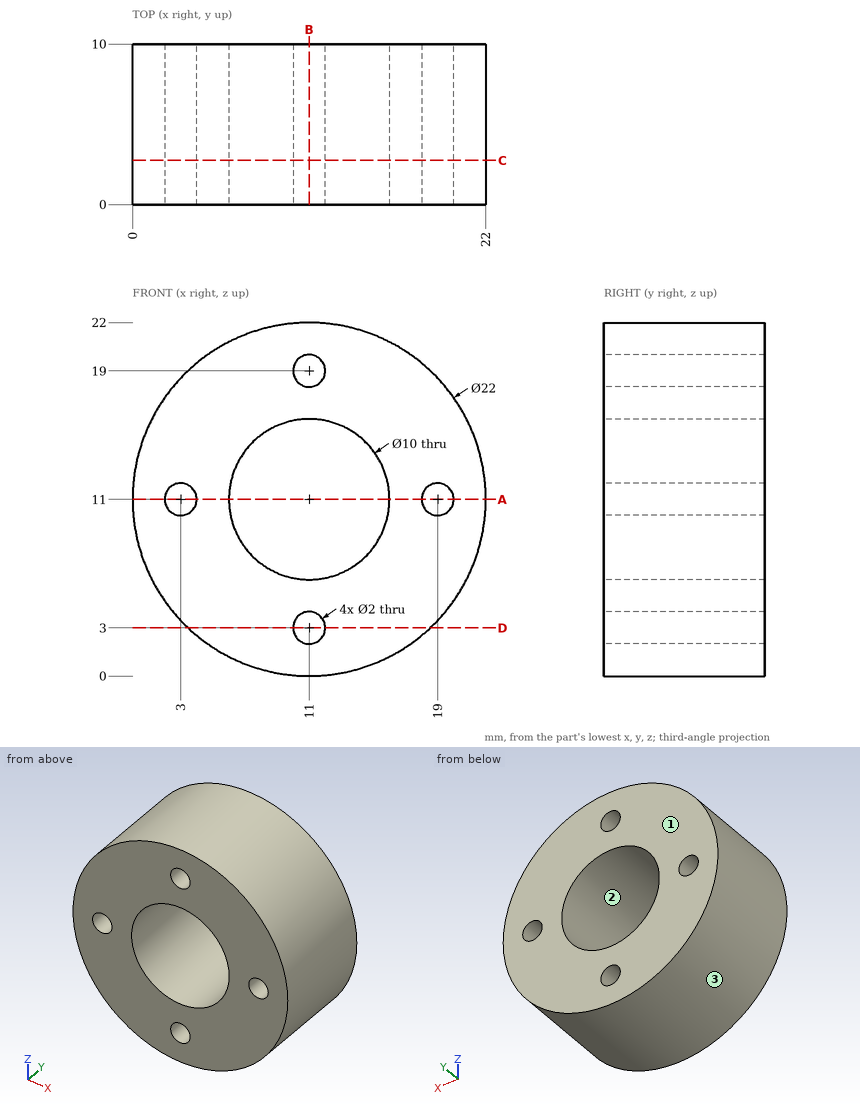
Verification items for this drawing (mm, ordinates from the low corner). Give positions to 0.01 mm unless a question says otherwise; leave off trailing zeros. Write each loop counter-clockwise with the first axis right and the second up, starting at its lowest first coordinate (ties: lowest second). Pieces come first, ordered by that corner, then holes. Notation, with made-up numbers: (-18.5, 27.5) - (1.5, 27.5) arc R19 cw to (1.5, 48.5) - close; hole circle Ø10 at (12, 74.5). An arc over 180 degrees is marked (long way). Answer as CSV lines item,"result". Start each with the question number.
1. Sectioned sample at B-B (x = 11). Record the boundary of the cut face in (y, z), then the cut area to 3 significant figures.
2. Thickness scan on line 1 (Z direction, x = 11, y = 4.75); line 2 (Z direction, x = 10.5, y = 5.25); line 3 (Z direction, x = 2.75, y = 8). Record the ranges inside material, lowest first.
3. Sectioned sample at A-A (z = 11). Record the boundary of the cut face in (x, y).
4. Sectioned sample at D-D (z = 3). Record the boundary of the cut face in (x, y).
5. Draft check along X on the marked faces 1, 2 and 3. Enter one of: pulls with the +X half, pulls with the -X half, needs draft (parallel to the pull), parting line crosses it, or undercut.
6. Depth check by flat-ended pin: pin 1 (2 mm diameter, centred on x = 17, y = 3.5, fed in from -Z); pin 2 (1 mm diameter, centred on y = 4, z = 16, fed in from -X); pin 3 (2 mm diameter, centred on y = 3.5, z = 12.5, fed in from +X). Enter the tip coordinate at first touch or a pass-through.
7. Sectioned sample at C-C (y = 2.75). Record the boundary of the cut face in (x, z), then the cut area to 3 significant figures.
Derived:
1,outline,"(0, 0) - (10, 0) - (10, 2) - (0, 2) - close; (0, 4) - (10, 4) - (10, 6) - (0, 6) - close; (0, 16) - (10, 16) - (10, 18) - (0, 18) - close; (0, 20) - (10, 20) - (10, 22) - (0, 22) - close"
1,area,"80.0 mm²"
2,line 1,"0 to 2, 4 to 6, 16 to 18, 20 to 22"
2,line 2,"0.01 to 2.13, 3.87 to 6.03, 15.97 to 18.13, 19.87 to 21.99"
2,line 3,"3.72 to 10.03, 11.97 to 18.28"
3,outline,"(0, 0) - (2, 0) - (2, 10) - (0, 10) - close; (4, 0) - (6, 0) - (6, 10) - (4, 10) - close; (16, 0) - (18, 0) - (18, 10) - (16, 10) - close; (20, 0) - (22, 0) - (22, 10) - (20, 10) - close"
4,outline,"(3.45, 0) - (10, 0) - (10, 10) - (3.45, 10) - close; (12, 0) - (18.55, 0) - (18.55, 10) - (12, 10) - close"
5,face 1,"needs draft"
5,face 2,"undercut"
5,face 3,"parting line crosses it"
6,pin 1,"z = 1.2"
6,pin 2,"x = 0.96"
6,pin 3,"x = 21.99"
7,outline,"circle Ø22 at (11, 11); hole circle Ø2 at (3, 11); hole circle Ø10 at (11, 11); hole circle Ø2 at (11, 3); hole circle Ø2 at (11, 19); hole circle Ø2 at (19, 11)"
7,area,"289 mm²"
